Here's the drawing with two shaded views (mm, measured from the low corner). I have some questions. A direction names the side the tool comes from. Coordinates: 2 decimals unless noted, no trailing zeros. Write each loop counter-clockwise with the first axis right and the second up, starting at its lowest first coordinate (ties: lowest second). Pieces come first, ordered by that corner, then holes. Notation, with made-up numbers: (75.5, 77.25) -> (80.5, 77.25) arc R27 ccw to (80.5, 114.25) -> close; hole circle Ø6 at (45.25, -6.75). An arc over 180 degrees is marked (long way). Put each result on its own line as item: value. Start each with the question number.
Item 1: For pin 1 (4 mm diameter, centred on x = 21.5, z = 37, fed in from -Y); pin 2 (1.5 mm diameter, centred on y = 20.5, z = 27.5, fed in from +X); pin 3 (1.5 mm diameter, centred on y = 39.5, z = 61.5, fed in from -X), each with a flat end and sliding along its axis, tell me the tip position at first contact or that it passes through.
Item 2: I want a section at B-B, the plane z = 60. List the corners of the cut face in (x, y) for me (1 decimal), then the cut area to 3 significant figures.
Item 3: On a 3-axis mill with a long thin cutter (end or side, diameter ignored), from which of +Z, -Z, +X, -X, +Y, -Y can I reach the whole of each face in a straight line? I mean the marked faces 4, 5 and 6. Say none if no direction works.
Item 4: I want a section at D-D, the plane y = 24.5. List the corners of the cut face in (x, z) for me, then the cut area to 3 significant figures.
Item 5: I want a section at C-C, the plane x = 36.5. List the corners of the cut face in (y, z) for me.
Item 6: I need wall thicknesses on line 1 (Z direction, x = 19, y = 37); line 2 (Y direction, x = 22, z = 22) (1 decimal); line 3 (Y direction, x = 14.5, z = 35). Which ranges of each line are inside material? Lowest first, please. Write a range as [from, to].
Item 7: I want a section at A-A, the plane z = 46.5. List the corners of the cut face in (x, y) for me, then the cut area to 3 significant figures.
Item 8: If we mould it in two halves opening along Y, with no side actions, what happens to the marked faces 1, 2 and 3? For each: released by +Y, released by -Y, zero draft, split by the parting line, or undercut.
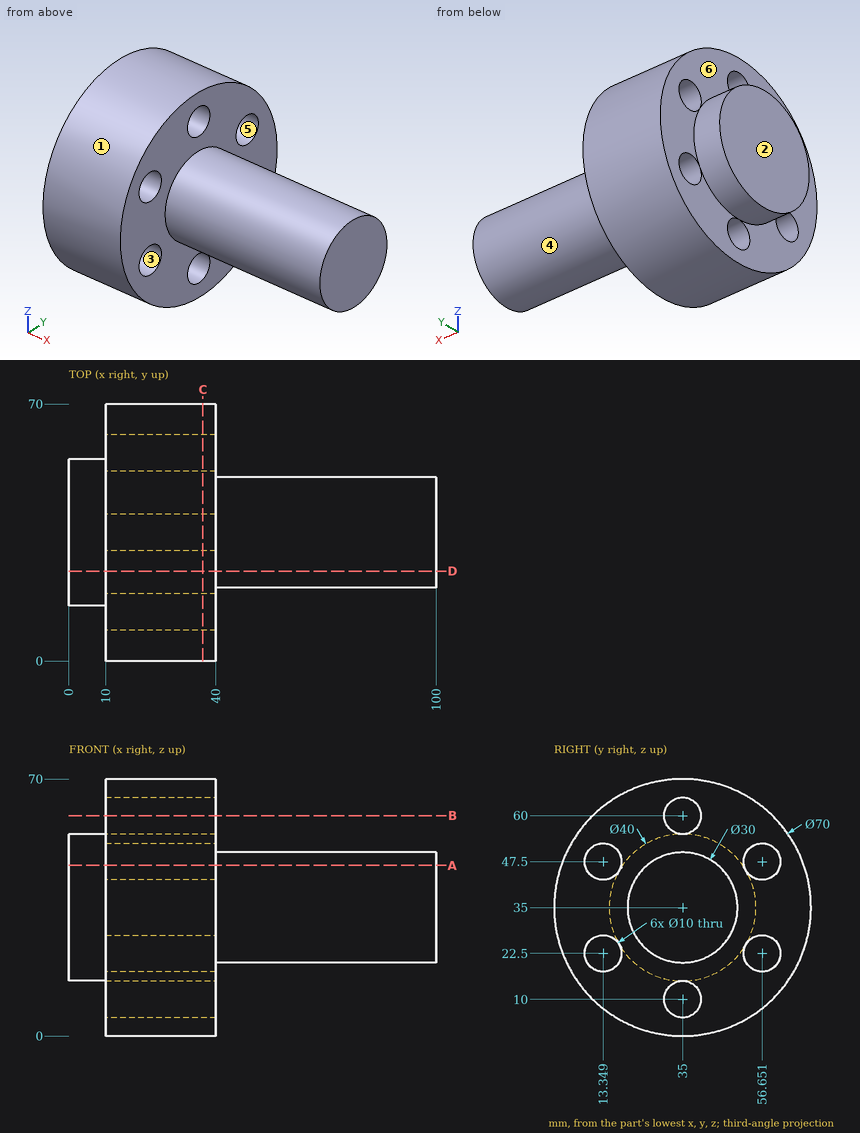
Calculated:
1. pin 1: stops at y = 0
1. pin 2: stops at x = 40
1. pin 3: stops at x = 10
2. outline: (10, 10.5) -> (40, 10.5) -> (40, 30) -> (10, 30) -> close; (10, 40) -> (40, 40) -> (40, 59.5) -> (10, 59.5) -> close
2. area: 1,170 mm2
3. face 4: +X
3. face 5: +X, -X
3. face 6: -X
4. outline: (0, 17.98) -> (10, 17.98) -> (10, 1.61) -> (40, 1.61) -> (40, 24.29) -> (100, 24.29) -> (100, 45.71) -> (40, 45.71) -> (40, 68.39) -> (10, 68.39) -> (10, 52.02) -> (0, 52.02) -> close
4. area: 3,630 mm2
5. outline: circle Ø70 at (35, 35); hole circle Ø10 at (13.35, 22.5); hole circle Ø10 at (13.35, 47.5); hole circle Ø10 at (35, 10); hole circle Ø10 at (35, 60); hole circle Ø10 at (56.65, 22.5); hole circle Ø10 at (56.65, 47.5)
6. line 1: z = [0.06, 5.42], [14.58, 55.42], [64.58, 69.94]
6. line 2: y = [2.5, 8.4], [18.3, 51.7], [61.6, 67.5]
6. line 3: y = [0, 70]
7. outline: (0, 18.64) -> (10, 18.64) -> (10, 18.25) -> (40, 18.25) -> (40, 25.37) -> (100, 25.37) -> (100, 44.63) -> (40, 44.63) -> (40, 51.75) -> (10, 51.75) -> (10, 51.36) -> (0, 51.36) -> close; (10, 1.94) -> (40, 1.94) -> (40, 8.45) -> (10, 8.45) -> close; (10, 61.55) -> (40, 61.55) -> (40, 68.06) -> (10, 68.06) -> close
7. area: 2,880 mm2
8. face 1: split by the parting line
8. face 2: zero draft
8. face 3: undercut
